Verification items for the finished model (mm, model axes). A direction names the side the tool comes from. Coordinates: 2 decimals unless noted, no trailing zeros. Write each loop counter-clockwise with the first axis right and the second up, starting at its lowest first coordinate (ties: lowest second). Pieces come first, ordered by that corner, then holes. Notation, with made-up numbers: M -27,80 L 3,80 A22 ccw 3,114 Z; hole C 70.25,-29 d9. An arc over 180 degrees is marked long. Answer in a Markdown table with one row per item.
from build123d import *

# Parameters (mm, degrees)
F0_R     = 7.5
F1_DEPTH = 3
F2_R     = 5
F3_R     = 5
F4_R     = 5
F5_R     = 5


# Not quite as in the source:
# - a feature of the source that left no trace in its solid (it failed there, or was rolled back) is left out


with BuildPart() as f1:
    # F0 (on Front) → F1 (new body)
    with BuildSketch(Plane.XZ):
        Polygon((-45.7000464201, 51.51183635), (-70.7000464201, 51.51183635), (-70.7000464201, 46.51183635), (-63.6224076152, 46.51183635), (-59.3452238418, 46.51183635), (-59.3452238418, 48.51183635), (-57.3452238418, 48.51183635), (-57.3452238418, 46.51183635), (-45.7000464201, 46.51183635), (-44.8452238418, 27.5310756076), (-57.3452238418, 27.5310756076), (-57.3452238418, 25.5310756076), (-59.3452238418, 25.5310756076), (-59.3452238418, 27.5310756076), (-69.8452238418, 27.5310756076), (-69.8452238418, 22.5310756076), (-44.8452238418, 22.5310756076), (-44.8452238418, -112.4689243924), (-29.8452238418, -112.4689243924), (-29.8452238418, -97.4689243924), (-25.8452238418, -97.4689243924), (-25.8452238418, -112.4689243924), (99.1547761582, -112.4689243924), (99.1547761582, -97.4689243924), (103.1547761582, -97.4689243924), (103.1547761582, -112.4689243924), (123.1547761582, -112.4689243924), (123.1547761582, -67.4689243924), (154.2856724769, -87.808891194), (155.0577331575, -86.6272304158), (123.2999535799, -63.48816365), (-20.7000464201, -63.48816365), (-20.7000464201, 51.51183635), (-30.7000464201, 51.51183635), (-30.7000464201, 61.51183635), (-35.7000464201, 61.51183635), (-35.7000464201, 51.51183635), (-40.7000464201, 51.51183635), (-40.7000464201, 61.51183635), (-45.7000464201, 61.51183635), align=None)
        with Locations((-7.8524835408, -88.0068540573)):
            Circle(F0_R, mode=Mode.SUBTRACT)
        with Locations((-31.9686569273, -43.2611815631)):
            Circle(F0_R, mode=Mode.SUBTRACT)
        with Locations((65.6582638621, -86.8446305394)):
            Circle(F0_R, mode=Mode.SUBTRACT)
        with Locations((-33.4214381874, 0)):
            Circle(F0_R, mode=Mode.SUBTRACT)
    extrude(amount=F1_DEPTH)

    # F2
    f2_edges = [f1.edges().sort_by_distance(p)[0] for p in [
        (-20.700046, -1.5, 51.511836),
    ]]
    fillet(f2_edges, radius=F2_R)

    # F3
    f3_edges = [f1.edges().sort_by_distance(p)[0] for p in [
        (123.154776, -1.5, -112.468924),
    ]]
    fillet(f3_edges, radius=F3_R)

    # F4
    f4_edges = [f1.edges().sort_by_distance(p)[0] for p in [
        (-44.845224, -1.5, -112.468924),
    ]]
    fillet(f4_edges, radius=F4_R)

    # F5
    f5_edges = [f1.edges().sort_by_distance(p)[0] for p in [
        (-20.700046, -1.5, -63.488164),
    ]]
    fillet(f5_edges, radius=F5_R)


solid = f1.part
1) Sectioned sample at B-B (x = 48). Record the cut outline in (y, z), then the cut area to 3 significant figures.
Response values:
| item | result |
|---|---|
| outline | M -3,-112.47 L 0,-112.47 L 0,-63.49 L -3,-63.49 Z |
| area | 147 mm² |
2) Release check for a two-part mould opening along X. For faces 3 (the face through (121.729, -1.521, -110.965)), 4 (the face through (-8.83, -1.48, -80.57)), 5 (the face through (17, -3, -64)) record: +X half, -X half, draft (parallel to the pull), parting line (faces both ways), or undercut.
Response values:
| item | result |
|---|---|
| face 3 | +X half |
| face 4 | undercut |
| face 5 | draft |
3) Depth check by flat-ended pin: pin 1 (0.9 mm diameter, centred on x = -67, y = -2, fed in from -Z); pin 2 (1.5 mm diameter, centred on x = -27.5, y = -1.5, fed in from -Z); pin 3 (0.6 mm diameter, centred on y = -2, z = 26, fed in from +X). Enter the tip coordinate at first touch or a pass-through.
Response values:
| item | result |
|---|---|
| pin 1 | stops at z = 22.53 |
| pin 2 | stops at z = -97.47 |
| pin 3 | stops at x = -20.7 |
4) Tool access check on faces 1 (the face through (-19.2, -1.52, -62.06)), 2 (the face through (138.502, -1.479, -77.497)). Record the directions out of +Z, -Z, +X, -X, +Y, -Y that give a thin tool (end or side, any length) a straight path to the whole face; none if there is none.
Response values:
| item | result |
|---|---|
| face 1 | +Z, +X, +Y, -Y |
| face 2 | -Z, +Y, -Y |
5) Thickness scan on L1, parallel to Z at x = -30.5, y = -2.1; L2, parallel to Z at x = -51.5, y = -0.2; L3, parallel to X at y = -2.2, z = 52. Record the ranges inside material, lowest first. Write a range as [from, to].
Response values:
| item | result |
|---|---|
| L1 | z = [-112.47, -50.62], [-35.91, -6.91], [6.91, 51.51] |
| L2 | z = [22.53, 27.53], [46.51, 51.51] |
| L3 | x = [-45.7, -40.7], [-35.7, -30.7] |
6) Sectioned sample at C-C (y = -1.6). Give the number of separate pieces and of enclosed holes in the cut face, then the cut area to 3 significant figures.
Response values:
| item | result |
|---|---|
| separate pieces | 1 |
| enclosed holes | 4 |
| area | 10,600 mm² |
7) Sectioned sample at D-D (z = 33). Record the cut outline in (x, y), then the cut area to 3 significant figures.
Response values:
| item | result |
|---|---|
| outline | M -45.09,-3 L -20.7,-3 L -20.7,0 L -45.09,0 Z |
| area | 73.2 mm² |
8) Sectioned sample at A-A (z = 0). Record the cut outline in (x, y).
Response values:
| item | result |
|---|---|
| outline | M -44.85,-3 L -40.92,-3 L -40.92,0 L -44.85,0 Z; M -25.92,-3 L -20.7,-3 L -20.7,0 L -25.92,0 Z |
